Check sheet for the drawn part. Datum: minimum x, y, z corner. Units: mm. Round coordinates to 2 decimals unless told otherwise and drop trailing zeros. Loops run counter-clockwise (first coordinate to the right, second up) from the corner with the lowest first, then second, coordinate; pieces in that order, holes last. Notation, with made-up numbers: (-36, 38) - (-21, 38) arc R18 cw to (-21, 68) - close; hole circle Ø1 at (-14, 18). An arc over 180 degrees is marked (long way). Use CSV: the item, a comma, the result in double quotes.
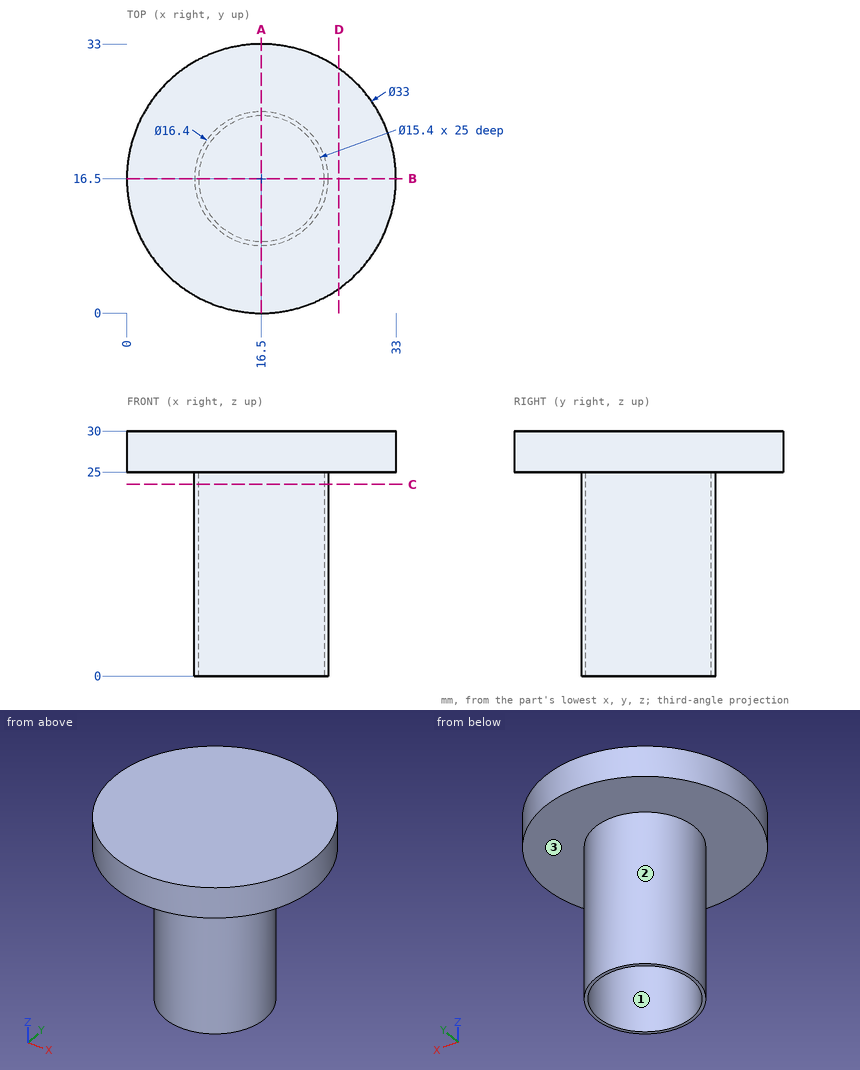
1) Mould release check, pull along X, two halves, no side actions. Record for the marked faces 1, 2 and 3: +X half, -X half, draft (parallel to the pull), parting line (faces both ways), or undercut.
Returned:
face 1,"undercut"
face 2,"parting line"
face 3,"draft"
2) Cross-section at C-C, the plane z = 23.5. Record the cut outline in (x, y), then the cut area to 3 significant figures.
Returned:
outline,"circle Ø16.4 at (16.5, 16.5); hole circle Ø15.4 at (16.5, 16.5)"
area,"25.0 mm²"
3) Cross-section at A-A, the plane x = 16.5. Record the cut outline in (y, z), then the cut area to 3 significant figures.
Returned:
outline,"(0, 25) - (8.3, 25) - (8.3, 0) - (8.8, 0) - (8.8, 25) - (24.2, 25) - (24.2, 0) - (24.7, 0) - (24.7, 25) - (33, 25) - (33, 30) - (0, 30) - close"
area,"190 mm²"
4) Gauge pin test, flat ends, axial feed: pin 1 Ø1 at (x, y) = (24.5, 26.5) entering from -Z; pin 2 Ø6 at (y, z) = (14, 8.5) entering from +X; pin 3 Ø2 at (y, z) = (10, 24.5) entering from +X; pin 4 Ø17 at (x, y) = (13, 19.5) entering from -Z. Record the tip position at first contact, or that the pin passes through.
Returned:
pin 1,"stops at z = 25"
pin 2,"stops at x = 24.7"
pin 3,"stops at x = 32.01"
pin 4,"stops at z = 0"
5) Cross-section at D-D, the plane x = 26. Record the cut outline in (y, z).
Returned:
outline,"(3.01, 25) - (29.99, 25) - (29.99, 30) - (3.01, 30) - close"
6) Thickness scan on probe 1 along Y at (x, z) = (16.5, 12); probe 2 along Z at (x, y) = (26.5, 25.5); probe 3 along Y at (x, z) = (11.5, 13.5). Record the ranges inside material, lowest first. Write a range as [from, to].
Returned:
probe 1,"y = [8.3, 8.8], [24.2, 24.7]"
probe 2,"z = [25, 30]"
probe 3,"y = [10, 10.64], [22.36, 23]"
